from build123d import *

# Parameters (mm, degrees)
SKETCH1_W           = 165
SKETCH1_H           = 22
BOSS_EXTRUDE1_DEPTH = 5
SKETCH2_W           = 10
SKETCH2_H           = 15
BOSS_EXTRUDE2_DEPTH = 5
SKETCH3_R           = 2.5
BOSS_EXTRUDE3_DEPTH = 22


with BuildPart() as part:
    # Sketch1 → Boss-Extrude1 (new body)
    with BuildSketch(Plane.XY):
        with Locations((82.5, 11)):
            Rectangle(SKETCH1_W, SKETCH1_H)
    extrude(amount=BOSS_EXTRUDE1_DEPTH)

    # Sketch2 → Boss-Extrude2 (add)
    with BuildSketch(Plane.ZY):
        with Locations((2.5, 29.5)):
            Rectangle(SKETCH2_W, SKETCH2_H)
    extrude(amount=-BOSS_EXTRUDE2_DEPTH)

    # Sketch3 → Boss-Extrude3 (add)
    with BuildSketch(Plane(origin=(0, 22, 0), x_dir=(1, 0, 0), z_dir=(0, 1, 0))):
        with Locations((0, -2.5)):
            Circle(SKETCH3_R)
    extrude(amount=-BOSS_EXTRUDE3_DEPTH)


solid = part.part
For this review, take the finished solid that the model builds, in its own axes (mm). A direction names the side the tool comes from. Round coordinates to 2 decimals unless told otherwise and drop trailing zeros. Order: outer loops, then holes, each group sorted by start corner. A loop starts at its lowest first (then second) coordinate and runs counter-clockwise, first axis right, second up. Notation, with made-up numbers: (27, 12) -> (36, 12) arc R23 ccw to (36, 35) -> close; hole circle Ø4 at (-2.5, 68.25). An arc over 180 degrees is marked (long way). Write item = value, one per line. Start each with the question number.
1) To check wall thickness, follow line 1 (Z direction, x = 136.5, y = 20.5); line 2 (Y direction, x = 43.5, z = 1). State the ranges of each line that lie inside material, in increasing order. Write a range as from..to.
2) Take a section at A-A on z = 2.5. State the section outline as (x, y) points, plus the area to 3 significant figures.
3) Tool access review of faces 1 (the face through (84, 22, 2)), 2 (the face through (165, 11, 2)), 3 (the face through (0, 30, 2)): name each direction out of +Z, -Z, +X, -X, +Y, -Y from which nothing blocks a thin tool from reaching the whole face with its end or side.
4) Insertion check: pin 1 (6 mm diameter, centred on x = 54.5, z = 5.5, fed in from -Y); pin 2 (1 mm diameter, centred on x = 32, y = 8.5, fed in from +Z); pin 3 (2 mm diameter, centred on x = -2, z = 3, fed in from +Y); pin 4 (3 mm diameter, centred on y = 31, z = 3, fed in from +X). Each pin has a flat end and moves straight along its axis. Give the tip position at first contact, or say it passes through.
5) Take a section at C-C on x = 135.5. State the section outline as (y, z) points, plus the area to 3 significant figures.
6) Take a section at B-B on y = 24.5. State the section outline as (x, z) points.
Verdict:
q1.line_1 = 0..5
q1.line_2 = 0..22
q2.outline = (-2.5, 0) -> (165, 0) -> (165, 22) -> (5, 22) -> (5, 37) -> (0, 37) -> (0, 22) -> (-2.5, 22) -> close
q2.area = 3,760 mm2
q3.face_1 = +Z, -Z, +X, +Y
q3.face_2 = +Z, -Z, +X, +Y, -Y
q3.face_3 = +Z, -Z, -X, +Y
q4.pin_1 = 0
q4.pin_2 = 5
q4.pin_3 = 22
q4.pin_4 = 5
q5.outline = (0, 0) -> (22, 0) -> (22, 5) -> (0, 5) -> close
q5.area = 110 mm2
q6.outline = (0, -2.5) -> (5, -2.5) -> (5, 7.5) -> (0, 7.5) -> close
